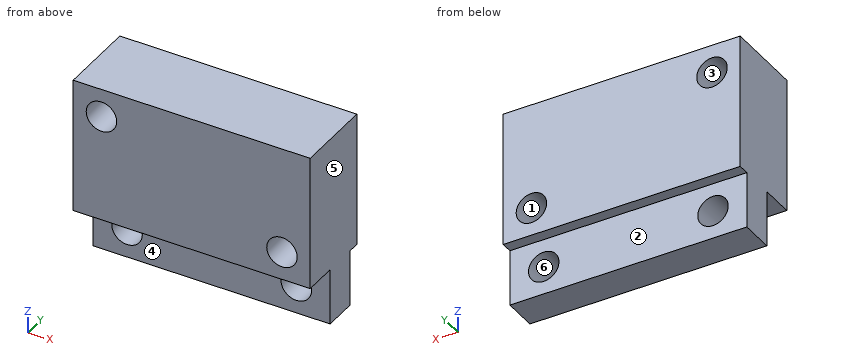
```python
from build123d import *

# Parameters (mm, degrees)
SKETCH1_W              = 21
SKETCH1_H              = 17
BOSS_EXTRUDE1_DEPTH    = 7
SKETCH2_W              = 21
SKETCH2_H              = 5
CUT_EXTRUDE1_DEPTH     = 1
M2_5_CLEARANCE_HOLE1_D = 2.7
SKETCH5_W              = 21
SKETCH5_H              = 5
CUT_EXTRUDE2_DEPTH     = 3
M2_5_CLEARANCE_HOLE2_D = 2.7


with BuildPart() as part:
    # Sketch1 → Boss-Extrude1 (new body)
    with BuildSketch(Plane(origin=(0, 0, 0), x_dir=(1, 0, 0), z_dir=(0, 1, 0))):
        Rectangle(SKETCH1_W, SKETCH1_H)
    extrude(amount=BOSS_EXTRUDE1_DEPTH)

    # Sketch2 → Cut-Extrude1 (cut)
    with BuildSketch(Plane(origin=(0, 7, 0), x_dir=(1, 0, 0), z_dir=(0, 1, 0))):
        with Locations((0, 6)):
            Rectangle(SKETCH2_W, SKETCH2_H)
    extrude(amount=-CUT_EXTRUDE1_DEPTH, mode=Mode.SUBTRACT)

    # M2.5 Clearance Hole1 (through all)
    with Locations(Plane(origin=(0, 7, 0), x_dir=(1, 0, 0), z_dir=(0, 1, 0))):
        with Locations((-8, -6), (8, 1)):
            Hole(M2_5_CLEARANCE_HOLE1_D / 2)

    # Sketch5 → Cut-Extrude2 (cut)
    with BuildSketch(Plane.XZ):
        with Locations((0, -6)):
            Rectangle(SKETCH5_W, SKETCH5_H)
    extrude(amount=-CUT_EXTRUDE2_DEPTH, mode=Mode.SUBTRACT)

    # M2.5 Clearance Hole2 (through all)
    with Locations(Plane(origin=(0, 3, 0), x_dir=(-1, 0, 0), z_dir=(0, -1, 0))):
        with Locations((-7.5, 6), (7.5, 6)):
            Hole(M2_5_CLEARANCE_HOLE2_D / 2)


solid = part.part
```
Read the model definition and answer for the solid it produces. Units are mm, in the model's axes. Face numbers are marked on the shaded views. A direction names the side the tool comes from. Give positions to 0.01 mm unless a question says otherwise; leave off trailing zeros. Order: outer loops, then holes, each group sorted by start corner. A loop starts at its lowest first (then second) coordinate and runs counter-clockwise, first axis right, second up. Notation, with made-up numbers: (23, -19.75) -> (31, -19.75) arc R23 cw to (31, 16.25) -> close; hole circle Ø9 at (-30.75, 12.5). An arc over 180 degrees is marked (long way). One line per item, written item: value. Start each with the question number.
(1) A tool of negligible diameter and unlimited length cuts with its end or side. For the marked faces 1 and 2, from which of +Z, -Z, +X, -X, +Y, -Y can it reach the whole face along a straight path? Write none if from no direction.
(2) The part is cut by section D-D (y = 6.5). Determine the outline of the cut face in (x, z).
(3) The part is cut by section A-A (y = 4.5). Determine the outline of the cut face in (x, z), and give its area (3 significant figures).
(4) The part is cut by section C-C (x = 7.75). Determine the outline of the cut face in (y, z), and give its area (3 significant figures).
(5) Flat-ended cylindrical pins translate along their axes: P1, Ø2.5, axis at x = -5, z = -6, coming from the +Y side; P2, Ø3.5, axis at x = -1.5, y = 1, coming from the -Z side; P3, Ø2.5, axis at x = 0.5, z = -6, coming from the -Y side. Find the tip coordinate at first contact, or state that the pin passes through.
(6) For a pull along X with two mould halves and no side action, classify the marked faces 3, 4, 5 and 6 as released by +X, released by -X, zero draft, split by the parting line, or undercut.
(7) The part is cut by section B-B (z = -1). Determine the outline of the cut face in (x, y), and give its area (3 significant figures).
(8) Straight lines are drawn through the part: L1, parallel to X at y = 3.8, z = -6; L2, parallel to Z at x = 7.5, y = 4.7; L3, parallel to Z at x = -7.5, y = 3.9. For each, find the intervals that lie inside material, in ascending order.
Taken from the geometry:
1. face 1: +Y, -Y
1. face 2: -Z, +X, -X, +Y
2. outline: (-10.5, -3.5) -> (10.5, -3.5) -> (10.5, 8.5) -> (-10.5, 8.5) -> close; hole circle Ø2.7 at (-8, 6); hole circle Ø2.7 at (8, -1)
3. outline: (-10.5, -8.5) -> (10.5, -8.5) -> (10.5, 8.5) -> (-10.5, 8.5) -> close; hole circle Ø2.7 at (-8, 6); hole circle Ø2.7 at (-7.5, -6); hole circle Ø2.7 at (7.5, -6); hole circle Ø2.7 at (8, -1)
3. area: 334 mm^2
4. outline: (0, -3.5) -> (3, -3.5) -> (3, -4.67) -> (6, -4.67) -> (6, -3.5) -> (7, -3.5) -> (7, -2.33) -> (0, -2.33) -> close; (0, 0.33) -> (7, 0.33) -> (7, 8.5) -> (0, 8.5) -> close; (3, -8.5) -> (6, -8.5) -> (6, -7.33) -> (3, -7.33) -> close
4. area: 72.5 mm^2
5. P1: y = 6
5. P2: z = -3.5
5. P3: y = 3
6. face 3: undercut
6. face 4: zero draft
6. face 5: released by +X
6. face 6: undercut
7. outline: (-10.5, 0) -> (6.65, 0) -> (6.65, 7) -> (-10.5, 7) -> close; (9.35, 0) -> (10.5, 0) -> (10.5, 7) -> (9.35, 7) -> close
7. area: 128 mm^2
8. L1: -10.5 to -8.85, -6.15 to 6.15, 8.85 to 10.5
8. L2: -8.5 to -7.35, -4.65 to -2.25, 0.25 to 8.5
8. L3: -8.5 to -7.35, -4.65 to 4.75, 7.25 to 8.5
